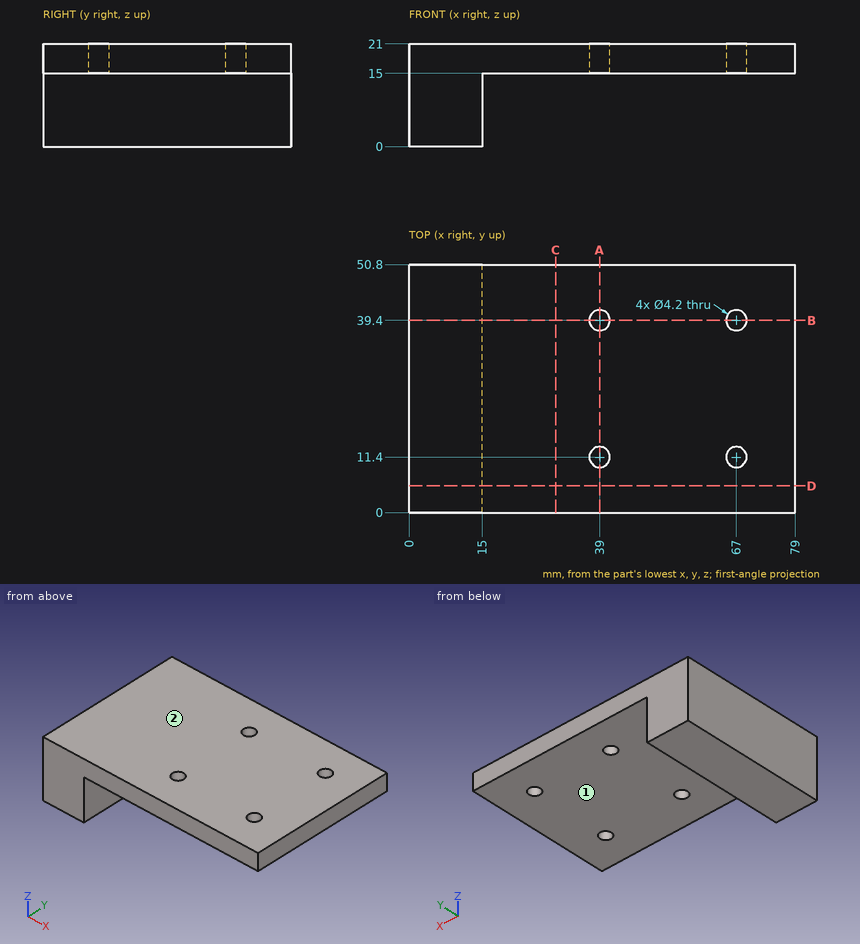
Design review of the part shown in the three views and the two pictorial views. Dimensions are in mm from the part's minimum x, y and z. A direction names the side the tool comes from. Give positions to 0.01 mm unless a question says otherwise; leave off trailing zeros. Write each loop counter-clockwise with the first axis right and the second up, starting at its lowest first coordinate (ties: lowest second). Pieces come first, ordered by that corner, then holes. Notation, with made-up numbers: (-24.75, 39.25) -> (22.25, 39.25) arc R29 cw to (22.25, 67.25) -> close; hole circle Ø4 at (6, -13). An arc over 180 degrees is marked (long way). Answer in a Markdown table with one row per item.
1) Add section D-D on y = 5.5. State the section outline as (x, z) points, plus the area to 3 significant figures.
Worked answers:
| item | result |
|---|---|
| outline | (0, 0) -> (15, 0) -> (15, 15) -> (79, 15) -> (79, 21) -> (0, 21) -> close |
| area | 699 mm² |
2) Clearance check with flat-ended pins moving along their axes: P1, Ø15, axis at x = 54, y = 38, coming from the -Z side; P2, Ø7.5, axis at y = 35, z = 7.5, coming from the +X side. State where each tip first meets the part, or that it passes through.
Worked answers:
| item | result |
|---|---|
| P1 | z = 15 |
| P2 | x = 15 |
3) For L1, parallel to Y at x = 39, z = 19.5; L2, parallel to Z at x = 19, y = 46.5; L3, parallel to X at y = 22, z = 2.5, list the stretches that pass through material, from the lowest coordinate up. Write a range as [from, to].
Worked answers:
| item | result |
|---|---|
| L1 | [0, 9.3], [13.5, 37.3], [41.5, 50.8] |
| L2 | [15, 21] |
| L3 | [0, 15] |
4) Add section B-B on y = 39.4. State the section outline as (x, z) points, plus the area to 3 significant figures.
Worked answers:
| item | result |
|---|---|
| outline | (0, 0) -> (15, 0) -> (15, 15) -> (36.9, 15) -> (36.9, 21) -> (0, 21) -> close; (41.1, 15) -> (64.9, 15) -> (64.9, 21) -> (41.1, 21) -> close; (69.1, 15) -> (79, 15) -> (79, 21) -> (69.1, 21) -> close |
| area | 649 mm² |
5) Add section A-A on x = 39. State the section outline as (y, z) points, plus the area to 3 significant figures.
Worked answers:
| item | result |
|---|---|
| outline | (0, 15) -> (9.3, 15) -> (9.3, 21) -> (0, 21) -> close; (13.5, 15) -> (37.3, 15) -> (37.3, 21) -> (13.5, 21) -> close; (41.5, 15) -> (50.8, 15) -> (50.8, 21) -> (41.5, 21) -> close |
| area | 254 mm² |
6) Add section C-C on x = 30. State the section outline as (y, z) points, plus the area to 3 significant figures.
Worked answers:
| item | result |
|---|---|
| outline | (0, 15) -> (50.8, 15) -> (50.8, 21) -> (0, 21) -> close |
| area | 305 mm² |
7) Tool access review of the marked faces 1 and 2: name each direction out of +Z, -Z, +X, -X, +Y, -Y from which nothing blocks a thin tool from reaching the whole face with its end or side.
Worked answers:
| item | result |
|---|---|
| face 1 | -Z, +X, +Y, -Y |
| face 2 | +Z, +X, -X, +Y, -Y |
